Autodesk Inventor part; units mm, degrees
ref_plane "YZ Plane" through (0, 0, 0) normal (1, 0, 0) x (0, 1, 0)
ref_plane "XZ Plane" through (0, 0, 0) normal (0, 1, 0) x (-1, 0, 0)
ref_plane "XY Plane" through (0, 0, 0) normal (0, 0, 1) x (1, 0, 0)
ref_plane "Work Plane1" through (0, 0, 0) normal (0, 0, 1) x (1, 0, 0)
sketch "Sketch1" plane through (0, 0, 0) normal (0, 0, 1) x (1, 0, 0)
  circle A0 centre (6.843, -28.9967) radius 1.4
  circle A1 centre (26.1569, -28.9967) radius 1.4
  circle A2 centre (26.1569, -23.9967) radius 1.4
  circle A3 centre (6.843, -23.9967) radius 1.4
  line L0 (0.4643, -12) -> (0, -12) construction
  line L1 (3.1567, -14.6923) -> (0.4643, -12) construction
  line L2 (3.1567, -32.6831) -> (3.1567, -14.6923) construction
  line L3 (10.5294, -32.6831) -> (3.1567, -32.6831)
  line L4 (10.5294, -14.6923) -> (10.5294, -32.6831) construction
  line L5 (9, -11) -> (10.5294, -14.6923) construction
  line L6 (2.8, -11) -> (9, -11) construction
  line L7 (2.8, 0) -> (2.8, -11) construction
  line L8 (30.2, 0) -> (2.8, 0) construction
  line L9 (30.2, 0) -> (30.2, -11) construction
  line L10 (24, -11) -> (30.2, -11) construction
  line L11 (24, -11) -> (22.4706, -14.6923) construction
  line L12 (22.4706, -14.6923) -> (22.4706, -32.6831) construction
  line L13 (22.4706, -32.6831) -> (29.8433, -32.6831)
  line L14 (29.8433, -32.6831) -> (29.8433, -14.6923) construction
  line L15 (29.8433, -14.6923) -> (32.5357, -12) construction
  line L16 (33, -12) -> (32.5357, -12) construction
  line L17 (33, -12) -> (33, 5) construction
  line L18 (0, 5) -> (0, -12) construction
  circle A4 centre (16.4744, -46.03) radius 10
  circle A5 centre (16.4744, -46.03) radius 12.5
  line L19 (31.4744, -31.03) -> (1.4744, -31.03) construction
  line L20 (1.4744, -31.03) -> (1.4744, -61.03) construction
  line L21 (1.4744, -61.03) -> (31.4744, -61.03) construction
  line L22 (31.4744, -61.03) -> (31.4744, -31.03) construction
  line L23 (31.4744, -31.03) -> (1.4744, -61.03) construction
  line L24 (1.4744, -31.03) -> (31.4744, -61.03) construction
  line L25 (31.4744, -61.03) -> (1.4744, -61.03)
  line L26 (1.4744, -61.03) -> (1.4744, -31.03)
  line L27 (1.4744, -31.03) -> (31.4744, -31.03)
  line L28 (31.4744, -31.03) -> (31.4744, -61.03)
  line L29 (31.4744, -61.03) -> (1.4744, -31.03) construction
  line L30 (1.4744, -61.03) -> (31.4744, -31.03) construction
  line L31 (1.4744, -31.03) -> (3.1567, -21.6555)
  line L32 (3.1567, -21.6555) -> (29.8433, -21.6555)
  line L33 (31.4744, -31.03) -> (29.8433, -21.6555)
  circle A6 centre (15.4444, 14.8) radius 2
  line L34 (19.4444, 18.8) -> (33, 5)
  line L35 (11.4444, 18.8) -> (19.4444, 18.8)
  line L36 (0, 5) -> (11.4444, 18.8)
  circle A7 centre (3.9444, 3.3) radius 1.45
  circle A8 centre (26.9444, 3.3) radius 1.45
  point P0 (0, 0)
  dimension "d0" = 25
  dimension "d1" = 30
  dimension "d2" = 30
extrude "Extrusion1" add sketch "Sketch1" along normal blind 5 contours L25 L26 L27 L28 | L27 L31 L32 L33
sketch "Sketch2" plane through (0, 0, 0) normal (0, 0, -1) x (-1, 0, 0)
  circle A0 centre (-16.4744, -46.03) radius 12.5
  circle A1 centre (-16.4744, -46.03) radius 10.5
  line L0 (0.4956, -63) -> (-33.4444, -63)
  circle A2 centre (-16.4744, -46.03) radius 12.5
  arc A3 (-23.9744, -56.03) -> (-8.9744, -56.03) centre (-16.4744, -46.03) ccw
  arc A4 (-21.3847, -34.5348) -> (-28.8847, -47.5252) centre (-16.4744, -46.03) ccw
  arc A5 (-4.0642, -47.5252) -> (-11.5642, -34.5348) centre (-16.4744, -46.03) ccw
  point P0 (0, 0)
  dimension "d5" = 21
extrude "Extrusion2" add sketch "Sketch2" against normal up to surface (5 mm away)
sketch "Sketch3" plane through (0, 0, 0) normal (0, 0, -1) x (-1, 0, 0)
  line L0 (-30.5357, -14) -> (-24, -14) construction
  line L1 (-30.5357, -14) -> (-29.8433, -14.6923) construction
  line L2 (-29.8433, -14.6923) -> (-29.8433, -32.6831) construction
  line L3 (-29.8433, -32.6831) -> (-22.4706, -32.6831)
  line L4 (-22.4706, -32.6831) -> (-10.5294, -32.6831)
  line L5 (-10.5294, -32.6831) -> (-10.5294, -22.0651)
  line L6 (-10.5294, -22.0651) -> (-22.4706, -22.0651)
  line L7 (-22.4706, -22.0651) -> (-22.4706, -32.6831)
  circle A0 centre (-6.843, -23.9967) radius 1.4 construction
  circle A1 centre (-26.1569, -23.9967) radius 1.4 construction
  circle A2 centre (-26.1569, -28.9967) radius 1.4 construction
  circle A3 centre (-6.843, -28.9967) radius 1.4 construction
  line L8 (-3.1567, -21.6555) -> (-1.4744, -31.03) construction
  line L9 (-29.8433, -21.6555) -> (-3.1567, -21.6555) construction
  line L10 (-31.4744, -31.03) -> (-29.8433, -21.6555) construction
  line L11 (-31.4744, -61.03) -> (-31.4744, -31.03) construction
  line L12 (-1.4744, -61.03) -> (-31.4744, -61.03)
  line L13 (-1.4744, -31.03) -> (-1.4744, -61.03) construction
  line L14 (-31.4744, -32.6831) -> (-29.8433, -32.6831)
  line L15 (-3.1567, -32.6831) -> (-1.4744, -32.6831)
  line L16 (-31.4744, -61.03) -> (-1.4744, -61.03)
  line L17 (-1.4744, -61.03) -> (-1.4744, -32.6831)
  line L18 (-1.4744, -32.6831) -> (-31.4744, -32.6831)
  line L19 (-31.4744, -32.6831) -> (-31.4744, -61.03)
  circle A4 centre (-26.1569, -28.9967) radius 1.4
  circle A5 centre (-26.1569, -23.9967) radius 1.4
  line L20 (-24, -14) -> (-24, -11)
  line L21 (-22.4706, -32.6831) -> (-22.4706, -14.6923)
  line L22 (-22.4706, -14.6923) -> (-24, -11)
  circle A6 centre (-16.4256, -45.91) radius 10.6939
  point P0 (0, 0)
extrude "Extrusion4" add sketch "Sketch3" along normal blind 5 contours L3 L4 L18 L15 L17 L12 L19 L14 | L7 L6 L5 L4
sketch "Sketch4" plane through (3.1567, -21.6555, 0) normal (0, 1, 0) x (1, 0, 0)
  line L0 (-6.8596, 8.2929) -> (32.2101, 8.2929)
  line L1 (32.2101, 8.2929) -> (32.2101, -9.1799)
  line L2 (32.2101, -9.1799) -> (-6.8596, -9.1799)
  line L3 (-6.8596, -9.1799) -> (-6.8596, 8.2929)
  point P0 (-3.1567, 0)
extrude "Extrusion5" cut sketch "Sketch4" against normal blind 1
sketch "Sketch5" plane through (0, 0, 5) normal (0, 0, 1) x (1, 0, 0)
  circle A0 centre (6.843, -28.9967) radius 1.4
  circle A1 centre (26.1569, -28.9967) radius 1.4
  line L0 (25.7553, -22.6555) -> (7.2447, -22.6555)
  arc A2 (6.4414, -22.6555) -> (7.2447, -22.6555) centre (6.843, -23.9967) ccw
  line L1 (6.4414, -22.6555) -> (2.9772, -22.6555)
  line L2 (2.9772, -22.6555) -> (1.4744, -31.03)
  line L3 (1.4744, -31.03) -> (1.4744, -61.03)
  line L4 (1.4744, -61.03) -> (31.4744, -61.03)
  line L5 (31.4744, -61.03) -> (31.4744, -31.03)
  line L6 (31.4744, -31.03) -> (30.0173, -22.6555)
  line L7 (30.0173, -22.6555) -> (26.5586, -22.6555)
  arc A3 (25.7553, -22.6555) -> (26.5586, -22.6555) centre (26.1569, -23.9967) ccw
  line L8 (10.5294, -20.3437) -> (22.4706, -20.3437)
  line L9 (22.4706, -20.3437) -> (22.4706, -24.9674)
  line L10 (22.4706, -24.9674) -> (10.5294, -24.9674)
  line L11 (10.5294, -24.9674) -> (10.5294, -20.3437)
  line L12 (10.5294, -22.6555) -> (22.4706, -22.6555)
  line L13 (10.5294, -20.3437) -> (22.4706, -24.9674) construction
  line L14 (22.4706, -20.3437) -> (10.5294, -24.9674) construction
  point P0 (0, 0)
  point P1 (16.5, -22.6555)
extrude "Extrusion6" cut sketch "Sketch5" against normal through all contours L9 L10 L11 L0 | L0 L11 L8 L9
ref_plane "Work Plane2" through (16.4744, -61.03, 5) normal (1, 0, 0) x (0, 0, -1)
sketch "Sketch6" plane through (16.4744, -61.03, 5) normal (1, 0, 0) x (0, 0, -1)
  line L0 (0, 5.17) -> (0.15, 5.17)
  line L1 (0, 5.17) -> (0.15, 5.17) construction
  line L2 (0.15, 5.17) -> (0.3567, 4.812)
  line L3 (0.3567, 4.812) -> (0.5067, 4.812)
  line L4 (0.5067, 4.812) -> (0.7133, 5.17)
  line L5 (0.7133, 5.17) -> (0.7133, 4.17)
  line L6 (0.7133, 4.17) -> (0, 4.17)
  line L7 (0, 4.17) -> (0, 5.17)
  line L8 (-2, 15.12) -> (12, 15.12)
  point P0 (5, 61.03)
  point P1 (0, 0)
  dimension "d16" = 0.15
  dimension "d17" = 0
  dimension "d18" = 120
  dimension "d19" = 0.15
  dimension "d20" = 120
  dimension "d21" = 1
  dimension "d22" = 0.7133
  dimension "d33" = 9.95
coil "Coil1" sketch "Sketch6" operation add axis through (16.4744, -45.91, 0) along (0, 0, -1) pitch 0.7133 turns 13 hand right
sketch "Sketch7" plane through (0, 0, 5) normal (0, 0, 1) x (1, 0, 0)
  circle A0 centre (16.4744, -46.03) radius 10.5
  circle A1 centre (16.4744, -46.03) radius 6
  point P0 (0, 0)
  point P1 (16.4744, -56.53)
  dimension "d34" = 12
extrude "Extrusion7" add sketch "Sketch7" against normal blind 0.3
sketch "Sketch8" plane through (0, 0, -5) normal (0, 0, -1) x (-1, 0, 0)
  circle A0 centre (-16.4256, -45.91) radius 10.6939
  circle A1 centre (-16.4256, -45.91) radius 8.8
  point P0 (0, 0)
  dimension "d37" = 17.6
extrude "Extrusion8" add sketch "Sketch8" against normal up to surface (9.7 mm away)
sketch "Sketch9" plane through (31.4744, -61.03, 5) normal (1, 0, 0) x (0, 0, -1)
  line L0 (0.3, 6.32) -> (0.3, 23.92)
  line L1 (10, 23.92) -> (10, 6.32)
  circle A0 centre (2.8356, 15.12) radius 1.45
  point P0 (5, 61.03)
  dimension "d40" = 2.9
extrude "Extrusion9" cut sketch "Sketch9" against normal through all
equation "\"d19\" = d16"
equation "\"d20\" = d18"
properties part number "30_Cube_Z_Focus_MGN_NEMA_adapter_M12"
CAD build for the part. Positions are in the model's coordinates, mm. A direction names the side the tool comes from. Round coordinates to 2 decimals unless told otherwise and drop trailing zeros. Write each loop counter-clockwise with the first axis right and the second up, starting at its lowest first coordinate (ties: lowest second). Pieces come first, ordered by that corner, then holes.
Item 1: Band-saw the part on A-A on x = 14. Write the cut outline in (y, z), then the cut area to 3 significant figures.
Filled in:
outline: (-61.03, -5) - (-54.37, -5) - (-54.37, 4.7) - (-51.5, 4.7) - (-51.5, 5) - (-61.03, 5) - close; (-40.56, 4.7) - (-37.45, 4.7) - (-37.45, -5) - (-24.97, -5) - (-24.97, 5) - (-40.56, 5) - close
area: 193 mm2
Item 2: Tool access for faces 4 (the flat face through (6.1, -27.6, 0)), 5 (the flat face through (22.471, -24, 3)), 6 (the flat face through (22.471, -29, -2)): list every direction of +Z, -Z, +X, -X, +Y, -Y with a clear straight run to the whole face (end or side of a thin tool).
Filled in:
face 4: -Z, -X, +Y
face 5: +Z, -Z, +Y
face 6: -Z, +X, +Y
Item 3: Band-saw the part on D-D on x = 23. Write the cut outline in (y, z).
Filled in:
outline: (-61.03, -5) - (-51.76, -5) - (-51.76, 4.7) - (-40.06, 4.7) - (-40.06, -5) - (-32.68, -5) - (-32.68, 0) - (-22.66, 0) - (-22.66, 5) - (-61.03, 5) - close
Item 4: Drop flat-ended pins along their axis: pin 1 Ø5 at (x, z) = (16, -0.5) entering from +Y; pin 2 Ø1.2 at (y, z) = (-24.5, 2) entering from -X; pin 3 Ø2.5 at (y, z) = (-45.91, 2.16) entering from -X; pin 4 Ø4 at (x, z) = (4, -3) entering from +Y. Give the stop position or say it passes through.
Filled in:
pin 1: stops at y = -24.97
pin 2: stops at x = 2.54
pin 3: passes through
pin 4: stops at y = -32.68
Item 5: Band-saw the part on B-B on y = -51.5. Write the cut outline in (x, z), then the cut area to 3 significant figures.
Filled in:
outline: (1.47, -5) - (9.63, -5) - (9.63, 4.7) - (14.01, 4.7) - (14.01, 5) - (1.47, 5) - close; (18.94, 4.7) - (23.22, 4.7) - (23.22, -5) - (31.47, -5) - (31.47, 5) - (18.94, 5) - close
area: 167 mm2
Item 6: Mould opens along X. For faces 1 (the flat face through (10, -46, 4.7)), 2 (the flat face through (30.756, -26.901, 2.465)), 3 (the flat face through (27, -32.683, -2)) say: released by +X, released by -X, zero draft, split by the parting line, or undercut.
Filled in:
face 1: undercut
face 2: released by +X
face 3: zero draft
Item 7: Band-saw the part on C-C on z = -2. Write the cut outline in (x, y).
Filled in:
outline: (1.47, -61.03) - (31.47, -61.03) - (31.47, -32.68) - (22.47, -32.68) - (22.47, -24.97) - (10.53, -24.97) - (10.53, -32.68) - (1.47, -32.68) - close; hole circle Ø17.6 at (16.43, -45.91)
Item 8: Drill centre lines: L1, parallel to Z at x = 3.5, y = -45.91; L2, parallel to Z at x = 23.5, y = -24.5; L3, parallel to Z at x = 10.5, y = -50. Where is each one in solid material? Low to high.
Filled in:
L1: z = -5 to 0.71, 3.61 to 5
L2: z = 0 to 5
L3: z = 4.7 to 5
